Part model, mm, in its own coordinate system. A direction names the side the tool comes from. Coordinates: 2 decimals unless noted, no trailing zeros. Write each loop counter-clockwise with the first axis right and the second up, starting at its lowest first coordinate (ties: lowest second). Pieces come first, ordered by that corner, then holes. Notation, with made-up numbers: (-15.5, -1) -> (-0.5, -1) arc R16 cw to (-0.5, 4) -> close; hole circle Ø6 at (-30.75, 43). An arc over 180 degrees is marked (long way). Write item = value, one per line.
from build123d import *

# Parameters (mm, degrees)
SKETCH10_W                     = 25
SKETCH10_H                     = 12.7
BOSS_EXTRUDE3_DEPTH            = 18
CBORE_FOR_M4_SHCS1_AT_2_COUNT  = 2
CBORE_FOR_M4_SHCS1_AT_2_PITCH  = 15
SKETCH19_W                     = 25
SKETCH19_H                     = 18
BOSS_EXTRUDE6_DEPTH            = 5
SKETCH20_W                     = 25
SKETCH20_H                     = 5
BOSS_EXTRUDE7_DEPTH            = 13.1
SKETCH21_W                     = 25
SKETCH21_H                     = 17.7
BOSS_EXTRUDE8_DEPTH            = 5
CUT_EXTRUDE1_DEPTH             = 33.885141021
CUT_EXTRUDE1_DEPTH_BACK        = 17.18
M3_CLEARANCE_HOLE6_D           = 3.4
M3_CLEARANCE_HOLE6_DEPTH       = 5
M3_CLEARANCE_HOLE6_CSINK_D     = 3.45
M3_CLEARANCE_HOLE6_CSINK_ANGLE = 90
M3_CLEARANCE_HOLE6_TIP         = 1.021463052
SKETCH27_W                     = 5.82
SKETCH27_H                     = 2.71
CUT_EXTRUDE2_DEPTH             = 5.82
SKETCH28_W                     = 5.82
SKETCH28_H                     = 2.71
CUT_EXTRUDE3_DEPTH             = 10.82


with BuildPart() as part:
    # Sketch10 → Boss-Extrude3 (new body)
    with BuildSketch(Plane(origin=(0, 0, 0), x_dir=(-1, 0, 0), z_dir=(0, 0, -1))):
        Rectangle(SKETCH10_W, SKETCH10_H)
    extrude(amount=-BOSS_EXTRUDE3_DEPTH)

    # Sketch17 → CBORE for M4 SHCS1 (revolve, cut)
    with BuildSketch(Plane(origin=(7.5, 0, 18), x_dir=(0, -1, 0), z_dir=(1, 0, 0))):
        Polygon((0, 0), (0, 18), (2.25, 18), (2.25, 4), (4, 4), (4, 0.025), (4.025, 0), align=None)
    cbore_for_m4_shcs1 = revolve(axis=Axis((7.5, 0, 24.35), (0, 0, -1)), mode=Mode.SUBTRACT)

    # CBORE for M4 SHCS1 at 2: CBORE for M4 SHCS1 ×2
    with Locations(*[(-i * CBORE_FOR_M4_SHCS1_AT_2_PITCH, 0, 0) for i in range(1, CBORE_FOR_M4_SHCS1_AT_2_COUNT)]):
        add(cbore_for_m4_shcs1, mode=Mode.SUBTRACT)

    # Sketch19 → Boss-Extrude6 (add)
    with BuildSketch(Plane(origin=(0, 6.35, 0), x_dir=(1, 0, 0), z_dir=(0, 1, 0))):
        with Locations((0, -9)):
            Rectangle(SKETCH19_W, SKETCH19_H)
    extrude(amount=BOSS_EXTRUDE6_DEPTH)

    # Sketch20 → Boss-Extrude7 (add)
    with BuildSketch(Plane(origin=(0, 0, 0), x_dir=(-1, 0, 0), z_dir=(0, 0, -1))):
        with Locations((0, 8.85)):
            Rectangle(SKETCH20_W, SKETCH20_H)
    extrude(amount=BOSS_EXTRUDE7_DEPTH)

    # Sketch21 → Boss-Extrude8 (add)
    with BuildSketch(Plane(origin=(0, 0, -13.1), x_dir=(-1, 0, 0), z_dir=(0, 0, -1))):
        with Locations((0, 2.5)):
            Rectangle(SKETCH21_W, SKETCH21_H)
    extrude(amount=BOSS_EXTRUDE8_DEPTH)

    # Sketch22 → Cut-Extrude1 (cut, two sides: drawn at the far end of the back side and taken through both)
    with BuildSketch(Plane(origin=(12.5, 0, 0), x_dir=(0, 0, -1), z_dir=(1, 0, 0)).offset(-CUT_EXTRUDE1_DEPTH_BACK)):
        with BuildLine():
            Line((104.872716508, 1.7), (18.1, 1.7))
            ThreePointArc((18.1, 1.7), (16.4, 0), (18.1, -1.7))
            Line((18.1, -1.7), (104.872716508, -1.7))
            Line((104.872716508, -1.7), (278.418149524, -1.7))
            Line((278.418149524, -1.7), (278.418149524, 1.7))
            Line((278.418149524, 1.7), (104.872716508, 1.7))
        make_face()
    extrude(amount=CUT_EXTRUDE1_DEPTH + CUT_EXTRUDE1_DEPTH_BACK, mode=Mode.SUBTRACT)

    # M3 Clearance Hole6
    with Locations(Plane(origin=(0, 0, -18.1), x_dir=(-1, 0, 0), z_dir=(0, 0, -1))):
        with Locations((8.59, 4.025), (8.59, -4.025)):
            CounterSinkHole(M3_CLEARANCE_HOLE6_D / 2, M3_CLEARANCE_HOLE6_CSINK_D / 2, depth=M3_CLEARANCE_HOLE6_DEPTH, counter_sink_angle=M3_CLEARANCE_HOLE6_CSINK_ANGLE)
            with Locations((0, 0, -(M3_CLEARANCE_HOLE6_DEPTH + M3_CLEARANCE_HOLE6_TIP / 2))):  # 118° drill point
                Cone(0, M3_CLEARANCE_HOLE6_D / 2, M3_CLEARANCE_HOLE6_TIP, mode=Mode.SUBTRACT)

    # Sketch27 → Cut-Extrude2 (cut)
    with BuildSketch(Plane.XZ.offset(6.35)):
        with Locations((-8.59, -15.6)):
            Rectangle(SKETCH27_W, SKETCH27_H)
    extrude(amount=-CUT_EXTRUDE2_DEPTH, mode=Mode.SUBTRACT)

    # Sketch28 → Cut-Extrude3 (cut)
    with BuildSketch(Plane(origin=(0, 11.35, 11.35), x_dir=(-1, 0, 0), z_dir=(0, 1, 0))):
        with Locations((8.59, -26.95)):
            Rectangle(SKETCH28_W, SKETCH28_H)
    extrude(amount=-CUT_EXTRUDE3_DEPTH, mode=Mode.SUBTRACT)


solid = part.part
Q1. Which spindle directions (+Z, -Z, +X, -X, +Y, -Y) get a long thin tool onto all of the face, cutting with end or side? Do faces 1 (the face through (6.299, -3.815, 16.015)), 2 (the face through (-9.843, 5.174, -17.507)), 3 (the face through (-11.5, -3, -16)), 4 (the face through (0, 6.35, -6)). Say none if no direction does.
Model answer:
face_1 = +Z
face_2 = -Z
face_3 = -Y
face_4 = +X, -X, -Y
Q2. Probe line 1 (Z direction, x = -6.5, y = -3) (3 decimals); line 2 (Y direction, x = -8.59, z = -13.55) (3 decimals); line 3 (Z direction, x = -11, y = 9) (3 decimals). List the from-to ranges inside material, lowest first. Write a range as from..to.
Model answer:
line_1 = -18.1..-16.955, -14.245..-13.1, 0..14
line_2 = -6.35..-5.725, -2.325..2.325, 5.725..11.35
line_3 = -18.1..-16.955, -14.245..18
Q3. Saw through at D-D on x = -1. Give the cut face in (y, z).
Model answer:
outline = (-6.35, -18.1) -> (-1.7, -18.1) arc R1.7 cw to (1.7, -18.1) -> (11.35, -18.1) -> (11.35, 18) -> (-6.35, 18) -> (-6.35, 0) -> (6.35, 0) -> (6.35, -13.1) -> (-6.35, -13.1) -> close
Q4. Pin check, flat tips, straight feed: pin 1 (3 mm diameter, centred on x = -8.59, y = 4.025, fed in from -Z); pin 2 (6.5 mm diameter, centred on x = 2, z = -6.5, fed in from -Y). Stop position of each tip, or through.
Model answer:
pin_1 = 0
pin_2 = 6.35
Q5. Saw through at C-C on y = 0. Count the separate pieces of the cut face and the enclosed holes in it, and give its area (3 significant figures).
Model answer:
separate_pieces = 4
enclosed_holes = 0
area = 356 mm²
Q6. Saw through at B-B on z = 4. Give the cut face in (x, y), and give its area (3 significant figures).
Model answer:
outline = (-12.5, -6.35) -> (12.5, -6.35) -> (12.5, 11.35) -> (-12.5, 11.35) -> close; hole circle Ø4.5 at (-7.5, 0); hole circle Ø4.5 at (7.5, 0)
area = 411 mm²
Q7. Mould opens along Z. For faces 5 (the face through (9, 2, 14)), 6 (the face through (-9.843, -2.876, -17.507)), 7 (the face through (-5.68, -3, -16)) say: released by +Z, released by -Z, zero draft, split by the parting line, or undercut.
Model answer:
face_5 = released by +Z
face_6 = zero draft
face_7 = undercut
Q8. Saw through at A-A on y = 8.5. Give the cut face in (x, z) (3 decimals), and give its area (3 significant figures).
Model answer:
outline = (-12.5, -18.1) -> (12.5, -18.1) -> (12.5, 18) -> (-12.5, 18) -> close; hole (-11.5, -16.955) -> (-5.68, -16.955) -> (-5.68, -14.245) -> (-11.5, -14.245) -> close
area = 887 mm²
